The model under review builds one solid part; all positions refer to its coordinate system, in mm. A direction names the side the tool comes from. Coordinates: 2 decimals unless noted, no trailing zeros. Write each loop counter-clockwise with the first axis right and the second up, starting at its lowest first coordinate (ties: lowest second). Pieces come first, ordered by that corner, then holes.
1) Add section D-D, the plane y = 192. State the section outline as (x, z) points (3 decimals), then the cut area to 3 significant figures.
2) For line 1 (Y direction, x = 0, z = 3) (3 decimals); line 2 (X direction, y = 125.5, z = 91.5) (3 decimals); line 3 (X direction, y = 117, z = 1) (3 decimals), list the stretches that pass through material, from the lowest coordinate up.
3) Mouldability with a two-part tool opening along X and no side actions: class faces 6 (the flat face through (115, 116, 184.882)), 7 (the flat face through (125.625, 116, 0)), 8 (the flat face through (-1, 118, -2.618)) as released by +X, released by -X, zero draft, split by the parting line, or undercut.
4) Add section C-C, the plane z = 2. State the section outline as (x, y) points (3 decimals).
5) For P1, Ø4, axis at x = -36, y = 147.5, coming from the +Z side; P2, Ø22.5, axis at x = 14, y = 132, coming from the +Z side, all flat-tipped, find the tip position at first contact; note any pin that passes through.
6) Machinability: for faces 1 (the flat face through (1, 29.375, 1)), 2 (the cylindrical face through (114.53, 103.14, -144.81)), 3 (the flat face through (1, 77, 9.832)), 4 (the cylindrical face through (-8.13, 80.89, 3.69)), 5 (the flat face through (103.125, 116, -72)), which of the approach directions +Z, -Z, +X, -X, +Y, -Y give a long, thin tool a straight path to every point of the face, cutting with its end or side? Answer none if there is none.
7) Add section B-B, the plane z = 142.5. State the section outline as (x, y) points (3 decimals), then the cut area to 3 significant figures.
8) Add section A-A, the plane y = 117.5. State the section outline as (x, z) points (3 decimals), then the cut area to 3 significant figures.
from build123d import *

# Parameters (mm, degrees)
BOSS_EXTRUDE2_DEPTH = 235
SKETCH2_R           = 50
CUT_EXTRUDE1_DEPTH  = 16.6
SKETCH4_R           = 50
CUT_EXTRUDE2_DEPTH  = 667.6
SCALE1_SCALE        = 0.75


with BuildPart() as part:
    # Sketch1 → Boss-Extrude2 (new body)
    with BuildSketch(Plane(origin=(0, 0, 0), x_dir=(1, 0, 0), z_dir=(0, 1, 0))):
        Polygon((-137.5, -243.4), (-167.5, -243.4), (-167.5, 243.4), (-137.5, 243.4), (-137.5, 10), (137.5, 10), (137.5, 243.4), (167.5, 243.4), (167.5, -243.4), (137.5, -243.4), (137.5, -10), (-137.5, -10), align=None)
    extrude(amount=BOSS_EXTRUDE2_DEPTH)

    # Sketch2 → Cut-Extrude1 (cut)
    with BuildSketch(Plane.XY.offset(10)):
        with Locations((0, 117.5)):
            Circle(SKETCH2_R)
    extrude(amount=-CUT_EXTRUDE1_DEPTH, mode=Mode.SUBTRACT)

    # Sketch4 → Cut-Extrude2 (cut)
    with BuildSketch(Plane(origin=(167.5, 0, 0), x_dir=(0, 0, -1), z_dir=(1, 0, 0))):
        with Locations((150, 117.5)):
            Circle(SKETCH4_R)
    extrude(amount=-CUT_EXTRUDE2_DEPTH, mode=Mode.SUBTRACT)


with BuildPart() as part_1:
    # Scale1: scaled about (0, 117.5, 9.327119411)
    add(part.part.scale(SCALE1_SCALE).moved(Location((0, 29.375, 2.331779853))))


solid = part_1.part
Geometry results:
1. outline: (-125.625, -180.218) - (-103.125, -180.218) - (-103.125, -5.168) - (103.125, -5.168) - (103.125, -180.218) - (125.625, -180.218) - (125.625, 184.882) - (103.125, 184.882) - (103.125, 9.832) - (-103.125, 9.832) - (-103.125, 184.882) - (-125.625, 184.882) - close
1. area: 19,500 mm2
2. line 1: y = 29.375 to 80, 155 to 205.625
2. line 2: x = -125.625 to -103.125, 103.125 to 125.625
2. line 3: x = -125.625 to -37.497, 37.497 to 125.625
3. face 6: zero draft
3. face 7: released by +X
3. face 8: undercut
4. outline: (-125.625, 29.375) - (125.625, 29.375) - (125.625, 205.625) - (-125.625, 205.625) - close; hole circle Ø75 at (0, 117.5)
5. P1: stops at z = 9.83
5. P2: stops at z = -2.62
6. face 1: +Z, -Z, +X, -X, -Y
6. face 2: +X, -X
6. face 3: +Z, +Y, -Y
6. face 4: +Z
6. face 5: -Z, +Y, -Y
7. outline: (-125.625, 29.375) - (-103.125, 29.375) - (-103.125, 205.625) - (-125.625, 205.625) - close; (103.125, 29.375) - (125.625, 29.375) - (125.625, 205.625) - (103.125, 205.625) - close
7. area: 7,930 mm2
8. outline: (-125.625, -180.218) - (-103.125, -180.218) - (-103.125, -147.668) - (-125.625, -147.668) - close; (-125.625, -72.668) - (-103.125, -72.668) - (-103.125, -5.168) - (103.125, -5.168) - (103.125, -72.668) - (125.625, -72.668) - (125.625, 184.882) - (103.125, 184.882) - (103.125, 9.832) - (37.5, 9.832) - (37.5, -2.618) - (-37.5, -2.618) - (-37.5, 9.832) - (-103.125, 9.832) - (-103.125, 184.882) - (-125.625, 184.882) - close; (103.125, -180.218) - (125.625, -180.218) - (125.625, -147.668) - (103.125, -147.668) - close
8. area: 15,200 mm2
